Autodesk Inventor part; units mm, degrees
ref_plane "YZ Plane" through (0, 0, 0) normal (1, 0, 0) x (0, 1, 0)
ref_plane "XZ Plane" through (0, 0, 0) normal (0, 1, 0) x (-1, 0, 0)
ref_plane "XY Plane" through (0, 0, 0) normal (0, 0, 1) x (1, 0, 0)
sketch "Szkic1" plane through (0, 0, 0) normal (1, 0, 0) x (0, 1, 0)
  circle A0 centre (0, 0) radius 16.5
  arc A1 (16.0869, 63.5) -> (15.2371, 62.2084) centre (20, 60) ccw construction
  arc A2 (-20.25, 65.244) -> (-15.2371, 62.2084) centre (-20, 60) ccw
  line L0 (20.25, 69.5) -> (-20.25, 69.5)
  line L1 (-20.25, 69.5) -> (-20.25, 65.244)
  line L2 (-20.25, 63.5) -> (-16.0869, 63.5) construction
  line L3 (20.25, 63.5) -> (20.25, 65.244) construction
  line L4 (16.0869, 63.5) -> (20.25, 63.5) construction
  line L5 (20.25, 65.244) -> (20.25, 69.5)
  line L6 (-20.25, 65.244) -> (-20.25, 63.5) construction
  line L7 (-16.0869, 63.5) -> (-13, 63.5) construction
  arc A3 (20.25, 65.244) -> (16.0869, 63.5) centre (20, 60) ccw construction
  arc A4 (-16.0869, 63.5) -> (-20.25, 65.244) centre (-20, 60) ccw construction
  line L8 (-15.2371, 62.2084) -> (-13, 63.5)
  line L9 (13, 63.5) -> (15.2371, 62.2084)
  arc A5 (15.2371, 62.2084) -> (20.25, 65.244) centre (20, 60) ccw
  line L10 (13, 63.5) -> (16.0869, 63.5) construction
  arc A6 (-15.2371, 62.2084) -> (-16.0869, 63.5) centre (-20, 60) ccw construction
  line L11 (-13, 63.5) -> (13, 63.5)
  line L12 (16.5, 0) -> (-16.5, 0) construction
  arc A7 (15.2371, -62.2084) -> (16.0869, -63.5) centre (20, -60) ccw construction
  arc A8 (-15.2371, -62.2084) -> (-20.25, -65.244) centre (-20, -60) ccw
  line L13 (20.25, -69.5) -> (-20.25, -69.5)
  line L14 (-20.25, -69.5) -> (-20.25, -65.244)
  line L15 (-20.25, -63.5) -> (-16.0869, -63.5) construction
  line L16 (20.25, -63.5) -> (20.25, -65.244) construction
  line L17 (16.0869, -63.5) -> (20.25, -63.5) construction
  line L18 (20.25, -65.244) -> (20.25, -69.5)
  line L19 (-20.25, -65.244) -> (-20.25, -63.5) construction
  line L20 (-16.0869, -63.5) -> (-13, -63.5) construction
  arc A9 (16.0869, -63.5) -> (20.25, -65.244) centre (20, -60) ccw construction
  arc A10 (-20.25, -65.244) -> (-16.0869, -63.5) centre (-20, -60) ccw construction
  line L21 (-15.2371, -62.2084) -> (-13, -63.5)
  line L22 (13, -63.5) -> (15.2371, -62.2084)
  arc A11 (20.25, -65.244) -> (15.2371, -62.2084) centre (20, -60) ccw
  line L23 (13, -63.5) -> (16.0869, -63.5) construction
  arc A12 (-16.0869, -63.5) -> (-15.2371, -62.2084) centre (-20, -60) ccw construction
  line L24 (-13, -63.5) -> (13, -63.5)
  line L25 (24.5, 75.5) -> (-19, 75.5)
  line L26 (-40, 75.5) -> (-40, -75.5)
  line L27 (-19, -75.5) -> (24.5, -75.5)
  line L28 (30.5, -69.5) -> (30.5, -31.5)
  arc A13 (30.5, 69.5) -> (24.5, 75.5) centre (24.5, 69.5) ccw
  arc A14 (24.5, -75.5) -> (30.5, -69.5) centre (24.5, -69.5) ccw
  line L29 (-40, 75.5) -> (-25, 75.5) construction
  line L30 (-25, 81.5) -> (-25, 94.5)
  line L31 (-31, 100.5) -> (-40, 100.5)
  line L32 (-40, 100.5) -> (-40, 75.5)
  arc A15 (-25, 94.5) -> (-31, 100.5) centre (-31, 94.5) ccw
  arc A16 (-25, 81.5) -> (-19, 75.5) centre (-19, 81.5) ccw
  line L33 (-40, -75.5) -> (-25, -75.5) construction
  line L34 (-25, -81.5) -> (-25, -94.5)
  line L35 (-31, -100.5) -> (-40, -100.5)
  line L36 (-40, -100.5) -> (-40, -75.5)
  arc A17 (-31, -100.5) -> (-25, -94.5) centre (-31, -94.5) ccw
  arc A18 (-19, -75.5) -> (-25, -81.5) centre (-19, -81.5) ccw
  line L37 (30.5, 25.5) -> (30.5, -25.5) construction
  line L38 (30.5, 31.5) -> (30.5, 69.5)
  line L39 (30.5, -31.5) -> (30.5, 31.5)
  circle A19 centre (0, 0) radius 18.5
  point P0 (-25, 100.5)
  point P1 (-25, -100.5)
  dimension "d0" = 33
  dimension "d1" = 10.5
  dimension "d3" = 20
  dimension "d4" = 60
  dimension "d6" = 6
  dimension "d8" = 3.5
  dimension "d9" = 150
  dimension "d10" = 150
  dimension "d11" = 26
  dimension "d12" = 13
  dimension "d13" = 6
  dimension "d14" = 6
  dimension "d15" = 10.5
  dimension "d16" = 20
  dimension "d17" = 6
  dimension "d18" = 15
  dimension "d19" = 25
  dimension "d20" = 6
  dimension "d21" = 15
  dimension "d22" = 25
  dimension "d23" = 6
  dimension "d50" = 37
  dimension "d55" = 40
  dimension "d56" = 0.25
  dimension "d57" = 0.25
extrude "Wyciągnięcie proste1" add sketch "Szkic1" along normal blind 45 contours A0 | L1 L0 L5 A5 L9 L11 L8 A2 | L21 L24 L22 A11 L18 L13 L14 A8 | A13 L38 L39 L28 A14 L27 A18 L34 A17 L35 L36 L26 L32 L31 A15 L30 A16 L25 | A19
extrude "Wyciągnięcie proste4" cut sketch "Szkic1" along normal through all contours A0 | L1 L0 L5 A5 L9 L11 L8 A2 | L21 L24 L22 A11 L18 L13 L14 A8
extrude "Wyciągnięcie proste7" cut sketch "Szkic1" along normal blind 7 contours A19
sketch "Szkic2" plane through (0, -25, 94.5) normal (0, 1, 0) x (1, 0, 0)
  circle A0 centre (37, 6.5) radius 5.5
  circle A1 centre (8, 6.5) radius 5.5
  circle A2 centre (37, 6.5) radius 3.25
  circle A3 centre (8, 6.5) radius 3.25
  line L0 (45, 13) -> (45, 0)
  line L1 (0, -6) -> (45, -6)
  line L2 (0, 13) -> (0, 0)
  point P0 (0, 94.5)
  dimension "d41" = 6.5
  dimension "d42" = 11
  dimension "d43" = 8
  dimension "d44" = 12.5
  dimension "d45" = 8
extrude "Wyciągnięcie proste5" cut sketch "Szkic2" against normal through all contours A2 | A3
extrude "Wyciągnięcie proste6" cut sketch "Szkic2" against normal blind 5
sketch "Szkic3" plane through (0, -19, 75.5) normal (0, 0, 1) x (1, 0, 0)
  line L0 (45, 32) -> (45, 6)
  line L1 (0, 32) -> (45, 32)
  line L2 (0, 6) -> (0, 32)
  line L3 (0, 6) -> (45, 6)
  line L4 (0, 6) -> (45, 6)
  line L5 (0, 32) -> (45, 6) construction
  line L6 (45, 32) -> (0, 6) construction
  circle A0 centre (22.5, 19) radius 3.25
  circle A1 centre (22.5, 19) radius 5.5
  point P0 (0, 19)
  dimension "d58" = 6.5
  dimension "d59" = 11
extrude "Wyciągnięcie proste9" cut sketch "Szkic3" against normal blind 60 contours A0
sketch "Szkic4" plane through (45, 0, 0) normal (1, 0, 0) x (0, 0, -1)
  line L0 (-35.5, 5.25) -> (-30, 5.25)
  line L1 (-30, 5.25) -> (-30, -5.25)
  line L2 (-30, -5.25) -> (-35.5, -5.25)
  line L3 (-35.5, -5.25) -> (-35.5, 5.25)
  line L4 (-75.5, 24.5) -> (-75.5, -19)
  point P0 (0, 0)
  dimension "d62" = 10.5
  dimension "d63" = 5.25
  dimension "d64" = 40
  dimension "d65" = 5.5
extrude "Wyciągnięcie proste10" cut sketch "Szkic4" against normal blind 28.75
mirror "Odbij3" about plane through (0, 0, 0) normal (0, 0, 1) of "Wyciągnięcie proste10", "Wyciągnięcie proste9", "Wyciągnięcie proste6", "Wyciągnięcie proste5"
sketch "Szkic5" plane through (0, 30.5, 69.5) normal (0, 1, 0) x (1, 0, 0)
  line L0 (0, 51) -> (0, 88)
  line L1 (0, 124.25) -> (0, 134.744)
  line L2 (0, -31) -> (0, 170)
  line L3 (0, 120) -> (13, 120)
  line L4 (13, 120) -> (13, 99)
  line L5 (13, 99) -> (0, 99)
  line L6 (0, 99) -> (0, 120)
  point P0 (0, 69.5)
  point P1 (0, 131.7084)
  point P2 (0, 99)
  dimension "d68" = 21
  dimension "d69" = 13
  dimension "d70" = 11
extrude "Wyciągnięcie proste11" cut sketch "Szkic5" against normal blind 18
sketch "Szkic6" plane through (13, 30.5, -50.5) normal (-1, 0, 0) x (0, 0, 1)
  line L0 (21, -18) -> (0, -18)
  line L1 (21, 0) -> (21, -18)
  line L2 (0, -18) -> (21, -18)
  line L3 (21, -18) -> (21, -10)
  line L4 (21, -10) -> (0, -10)
  line L5 (0, -10) -> (0, -18)
  point P0 (50.5, -30.5)
  dimension "d74" = 8
extrude "Wyciągnięcie proste12" cut sketch "Szkic6" against normal through all
sketch "Szkic7" plane through (0, 12.5, 69.5) normal (0, 1, 0) x (1, 0, 0)
  circle A0 centre (8.5, 114.5) radius 1.75
  circle A1 centre (8.5, 104.5) radius 1.75
  line L0 (0, 120) -> (13, 120)
  line L1 (0, 99) -> (0, 120)
  point P0 (0, 69.5)
  dimension "d77" = 5.5
  dimension "d78" = 10
  dimension "d79" = 3.5
  dimension "d80" = 8.5
extrude "Wyciągnięcie proste13" cut sketch "Szkic7" against normal through all
sketch "Szkic10" plane through (0, 0, 0) normal (-1, 0, 0) x (0, 0, 1)
  line L0 (-46.75, 12.5) -> (-43.25, 12.5)
  line L1 (-36.75, 12.5) -> (-33.25, 12.5)
  line L2 (-48, 6) -> (-42, 6)
  line L3 (-42, 6) -> (-42, 3.4)
  line L4 (-42, 3.4) -> (-48, 3.4)
  line L5 (-48, 3.4) -> (-48, 6)
  line L6 (-38, 6) -> (-32, 6)
  line L7 (-32, 6) -> (-32, 3.4)
  line L8 (-32, 3.4) -> (-38, 3.4)
  line L9 (-38, 3.4) -> (-38, 6)
  line L10 (-29.5, 12.5) -> (-50.5, 12.5)
  line L11 (-50.5, 12.5) -> (-50.5, 30.5)
  point P0 (0, 0)
  dimension "d83" = 6.5
  dimension "d84" = 2.6
  dimension "d85" = 6
  dimension "d86" = 6
  dimension "d87" = 2.5
  dimension "d89" = 10
extrude "Wyciągnięcie proste14" cut sketch "Szkic10" against normal blind 11
equation "\"d14\" = d13"
properties part number "XFloating" material "Tworzywo sztuczne ABS"
Design review of the part built by this model. Coordinates are the model's own, in mm. A direction names the side the tool comes from. Give positions to 0.01 mm unless a question says otherwise; leave off trailing zeros. Write each loop counter-clockwise with the first axis right and the second up, starting at its lowest first coordinate (ties: lowest second). Pieces come first, ordered by that corner, then holes. Notation, with made-up numbers: (47, 1.5) -> (86, 1.5) arc R30 ccw to (86, 40.5) -> close; hole circle Ø7 at (7.5, 19). An arc over 180 degrees is marked (long way). Answer in a Markdown table with one row per item.
(1) Consider section C-C (y = 0). Count the separate pieces of the cut face and the enclosed holes in it, then the cut area to 3 significant figures.
Results:
| item | result |
|---|---|
| separate pieces | 10 |
| enclosed holes | 2 |
| area | 3,790 mm2 |
(2) For faces 5 (the flat face through (31, 5.25, 33)), 6 (the flat face through (5, 3.4, -35)), 7 (the flat face through (22, -25, 88)), 8 (the cylindrical face through (36.284, -27.465, -93.453)), 9 (the flat face through (13, 26, -40)), list the 3-axis set-ups (+Z, -Z, +X, -X, +Y, -Y) from which the entire face can be reached by the end or side of a thin tool; tool diameter is ignored.
Results:
| item | result |
|---|---|
| face 5 | +X |
| face 6 | -X |
| face 7 | +Z, +X, -X, +Y |
| face 8 | +Y |
| face 9 | -X, +Y |
(3) Mouldability with a two-part tool opening along X and no side actions: class faces 1 (the flat face through (7, -17, 0)), 2 (the flat face through (16.25, 0, 33)), 3 (the flat face through (12, -30, 88)), 4 (the flat face through (22, -25, -88)) as +X half, -X half, draft (parallel to the pull), parting line (faces both ways), or undercut.
Results:
| item | result |
|---|---|
| face 1 | -X half |
| face 2 | +X half |
| face 3 | undercut |
| face 4 | draft |
(4) Clearance check with flat-ended pins moving along their axes: pin 1 (8 mm diameter, centred on x = 30.5, y = 15, fed in from +Z); pin 2 (1 mm diameter, centred on y = -26.5, z = -54.5, fed in from -X); pin 3 (6.5 mm diameter, centred on x = 7.5, z = -44, fed in from +Y); pin 4 (8 mm diameter, centred on y = 24, z = -44, fed in from -X). State where each tip first meets the part, or that it passes through.
Results:
| item | result |
|---|---|
| pin 1 | z = 75.5 |
| pin 2 | x = 0 |
| pin 3 | y = 12.5 |
| pin 4 | x = 13 |
(5) Consider section A-A (z = -88). State the section outline as (x, y) points.
Results:
| item | result |
|---|---|
| outline | (0, -40) -> (4.75, -40) -> (4.75, -30) -> (2.5, -30) -> (2.5, -25) -> (0, -25) -> close; (11.25, -40) -> (33.75, -40) -> (33.75, -30) -> (31.5, -30) -> (31.5, -25) -> (13.5, -25) -> (13.5, -30) -> (11.25, -30) -> close; (40.25, -40) -> (45, -40) -> (45, -25) -> (42.5, -25) -> (42.5, -30) -> (40.25, -30) -> close |
(6) Consider section B-B (z = 0). State the section outline as (x, y) points.
Results:
| item | result |
|---|---|
| outline | (0, -40) -> (45, -40) -> (45, -16.5) -> (7, -16.5) -> (7, -18.5) -> (0, -18.5) -> close; (0, 18.5) -> (7, 18.5) -> (7, 16.5) -> (45, 16.5) -> (45, 30.5) -> (0, 30.5) -> close |
(7) To check wall thickness, follow probe 1 along X at (y, z) = (-33, -88); probe 2 along Y at (x, z) = (22, -19); probe 3 along Y at (x, z) = (30, 0). State the ranges of each line that lie inside material, in increasing order.
Results:
| item | result |
|---|---|
| probe 1 | 0 to 4.75, 11.25 to 33.75, 40.25 to 45 |
| probe 2 | -40 to -3.21, 3.21 to 30.5 |
| probe 3 | -40 to -16.5, 16.5 to 30.5 |
